Drawing for the job (mm, zero at the part's lowest x, y, z). A direction names the side the tool comes from. Coordinates: 2 decimals unless noted, no trailing zeros. Write each loop counter-clockwise with the first axis right and the second up, starting at its lowest first coordinate (ties: lowest second). Pieces come first, ordered by that corner, then holes. Notation, with made-up numbers: (45.25, 30.5) -> (85.25, 30.5) arc R35 cw to (85.25, 68.5) -> close; hole circle Ø5 at (-10, -1.5). An arc over 180 degrees is marked (long way). Answer as CSV lines item,"result".
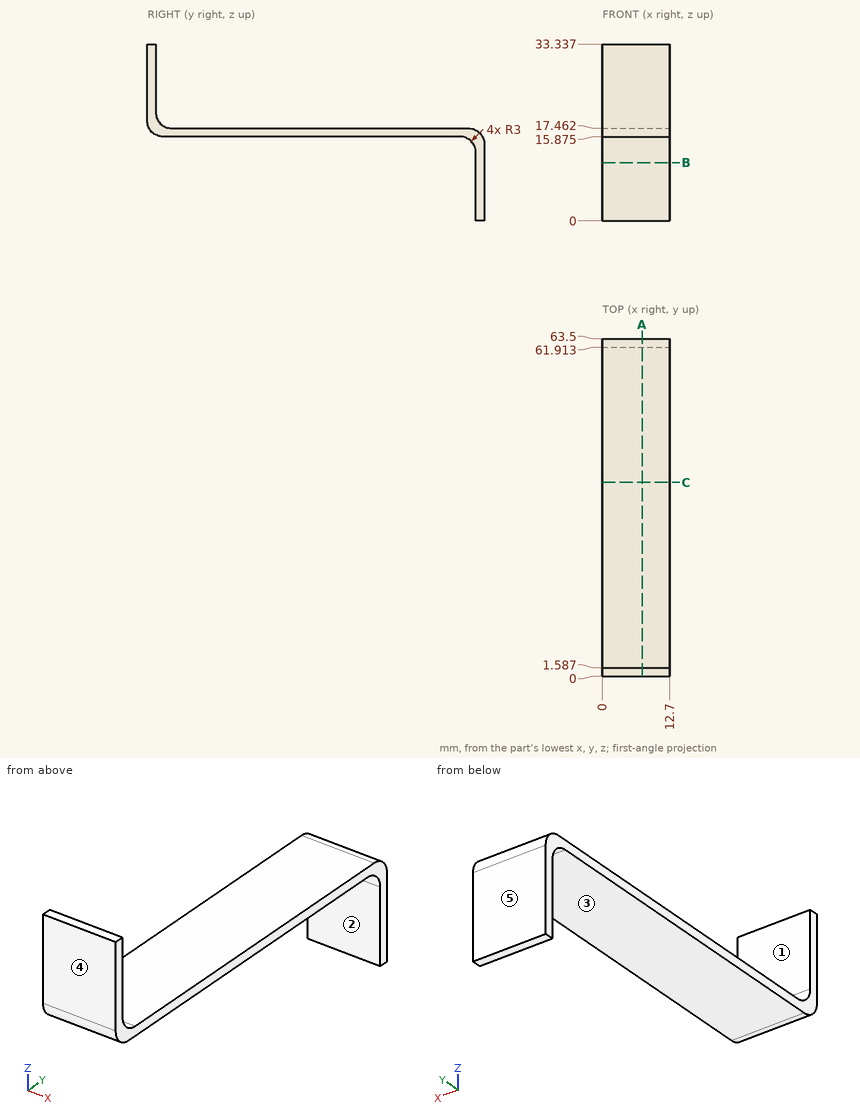
Item 1: Flat gauge pins, fed straight in: pin 1 (2 mm diameter, centred on x = 7.5, z = 16.5, fed in from +Y) (1 decimal); pin 2 (6.5 mm diameter, centred on x = 6, y = 36.5, fed in from -Z) (1 decimal); pin 3 (1 mm diameter, centred on x = 9, z = 13, fed in from -Y). Where does each tip first touch, or does it go through?
Answer below:
pin 1,"stops at y = 63.3"
pin 2,"stops at z = 15.9"
pin 3,"stops at y = 61.85"
Item 2: 3-axis set-ups, long thin cutter, end or side, ignore diameter. For the marked faces 1 and 2: which of +Z, -Z, +X, -X, +Y, -Y reach the whole face in a straight line?
Answer below:
face 1,"+Z, +X, -X, +Y"
face 2,"-Z, +X, -X, -Y"
Item 3: Wall check: line 1 (Y direction, x = 1.25, z = 20.5); line 2 (Y direction, x = 10.5, z = 7); line 3 (Z direction, x = 11.75, y = 19) (1 decimal). Give the ranges that are in metal, low to high. Write a range as from..to.
Answer below:
line 1,"y = 0..1.59"
line 2,"y = 61.91..63.5"
line 3,"z = 15.9..17.5"
Item 4: Saw through at C-C on y = 36.5. Give the cut face in (x, z) (1 decimal).
Answer below:
outline,"(0, 15.9) -> (12.7, 15.9) -> (12.7, 17.5) -> (0, 17.5) -> close"
Item 5: Saw through at A-A on x = 7.5. Give the cut face in (y, z) (1 decimal).
Answer below:
outline,"(0, 18.9) arc R3 ccw to (3, 15.9) -> (58.9, 15.9) arc R3 cw to (61.9, 12.9) -> (61.9, 0) -> (63.5, 0) -> (63.5, 14.5) arc R3 ccw to (60.5, 17.5) -> (4.6, 17.5) arc R3 cw to (1.6, 20.5) -> (1.6, 33.3) -> (0, 33.3) -> close"
Item 6: Saw through at B-B on z = 11. Give the cut face in (x, y).
Answer below:
outline,"(0, 61.91) -> (12.7, 61.91) -> (12.7, 63.5) -> (0, 63.5) -> close"
Item 7: Two-plate mould, pull along Y, no slides. Class the marked faces 3, 4 and 5: pulls with the +Y half, pulls with the -Y half, needs draft (parallel to the pull), parting line crosses it, or undercut.
Answer below:
face 3,"needs draft"
face 4,"pulls with the -Y half"
face 5,"pulls with the +Y half"
